Source: CAD feature listing. Evaluate the final solid. Frame: model axes, mm. A direction names the side the tool comes from. Round coordinates to 2 decimals unless told otherwise and drop trailing zeros. Loops run counter-clockwise (first coordinate to the right, second up) from the corner with the lowest first, then second, coordinate; pieces in that order, holes last.
(1) Section B-B, the plane x = 0. Return the cut outline in (y, z).
(2) Section D-D, the plane y = 20. Return the cut outline in (x, z), plus the area to 3 significant figures.
(3) Set-up query: faces 4 (the flat face through (49, -1, 15)), 5 (the cylindrical face through (48.85, -0.7, 1.57)). Return all of +Z, -Z, +X, -X, +Y, -Y with unobstructed straight access to the full face (end or side cutting, diameter ignored); none if empty.
(4) Section C-C, the plane y = -33. Return the cut outline in (x, z).
(5) Mould query, pull axis Y, two halves, no side actions, for faces 1 (the flat face through (-1, 1, 1.5)), 2 (the flat face through (0, -50, 1)), 3 (the cylindrical face through (0.65, -35.93, 0.74)). Classes: pulls with the +Y half, pulls with the -Y half, needs draft (parallel to the pull), parting line crosses it, or undercut.
(6) First-contact query: pin 1 Ø8 at (x, y) = (0, -33) entering from +Z. Flat tip, straight axial feed; report the tip coordinate or a pass-through.
(7) Material intervals for probe 1 along Y at (x, z) = (0, 0.6); probe 2 along X at (y, z) = (-10.5, 14); probe 3 along Z at (x, y) = (-2, 24), sorted ascending.
(8) Section A-A, the plane z = 20.5. Return the cut outline in (x, y).
```python
from build123d import *

# Parameters (mm, degrees)
SKETCH1_W                = 90
SKETCH1_H                = 100
BOSS_EXTRUDE1_DEPTH      = 10
CONVERT_SOLID1_START     = 1.5
CONVERT_SOLID1_OUTLINE_W = 90
CONVERT_SOLID1_OUTLINE_H = 100
CONVERT_SOLID1_DEPTH     = 8.5
EDGE_FLANGE1_DEPTH       = 100
EDGE_FLANGE2_DEPTH       = 100
SKETCH12_R               = 3
CUT_EXTRUDE1_DEPTH       = 75.849849699


# Read off the part's stored shape, not the designer's step: Convert-Solid1
# Sheet-metal steps are written as plain solids
with BuildPart() as part:
    # Sketch1 → Boss-Extrude1 (new body)
    with BuildSketch(Plane.XY):
        Rectangle(SKETCH1_W, SKETCH1_H)
    extrude(amount=BOSS_EXTRUDE1_DEPTH)

    # Convert-Solid1 outline → Convert-Solid1 (cut)
    with BuildSketch(Plane.XY.offset(CONVERT_SOLID1_START)):
        Rectangle(CONVERT_SOLID1_OUTLINE_W, CONVERT_SOLID1_OUTLINE_H)
    extrude(amount=CONVERT_SOLID1_DEPTH, mode=Mode.SUBTRACT)

    # Edge-Flange1 section (across the edge) → Edge-Flange1 (add)
    with BuildSketch(Plane(origin=(-49, 50, 1.5), x_dir=(1, 0, 0), z_dir=(0, -1, 0))):
        with BuildLine():
            Line((-1.5, 4), (-1.5, 22))
            Line((-1.5, 22), (0, 22))
            Line((0, 22), (0, 4))
            ThreePointArc((0, 4), (1.171572875, 1.171572875), (4, 0))
            Line((4, 0), (4, -1.5))
            ThreePointArc((4, -1.5), (0.110912703, 0.110912703), (-1.5, 4))
        make_face()
    extrude(amount=EDGE_FLANGE1_DEPTH)

    # Edge-Flange2 section (across the edge) → Edge-Flange2 (add)
    with BuildSketch(Plane(origin=(49, -50, 1.5), x_dir=(-1, 0, 0), z_dir=(0, 1, 0))):
        with BuildLine():
            Line((-1.5, 4), (-1.5, 22))
            Line((-1.5, 22), (0, 22))
            Line((0, 22), (0, 4))
            ThreePointArc((0, 4), (1.171572875, 1.171572875), (4, 0))
            Line((4, 0), (4, -1.5))
            ThreePointArc((4, -1.5), (0.110912703, 0.110912703), (-1.5, 4))
        make_face()
    extrude(amount=EDGE_FLANGE2_DEPTH)

    # Sketch12 → Cut-Extrude1 (cut, through all)
    with BuildSketch(Plane(origin=(0, 0, 0), x_dir=(-1, 0, 0), z_dir=(0, 0, -1))):
        with Locations((0, 33)):
            Circle(SKETCH12_R)
        with Locations((0, -33)):
            Circle(SKETCH12_R)
    extrude(amount=-CUT_EXTRUDE1_DEPTH, mode=Mode.SUBTRACT)


solid = part.part
```
Output values:
1. outline: (-50, 0) - (-36, 0) - (-36, 1.5) - (-50, 1.5) - close; (-30, 0) - (30, 0) - (30, 1.5) - (-30, 1.5) - close; (36, 0) - (50, 0) - (50, 1.5) - (36, 1.5) - close
2. outline: (-50.5, 5.5) arc R5.5 ccw to (-45, 0) - (45, 0) arc R5.5 ccw to (50.5, 5.5) - (50.5, 23.5) - (49, 23.5) - (49, 5.5) arc R4 cw to (45, 1.5) - (-45, 1.5) arc R4 cw to (-49, 5.5) - (-49, 23.5) - (-50.5, 23.5) - close
2. area: 211 mm2
3. face 4: +Z, +Y, -Y
3. face 5: -Z, +X, +Y, -Y
4. outline: (-50.5, 5.5) arc R5.5 ccw to (-45, 0) - (-3, 0) - (-3, 1.5) - (-45, 1.5) arc R4 cw to (-49, 5.5) - (-49, 23.5) - (-50.5, 23.5) - close; (3, 0) - (45, 0) arc R5.5 ccw to (50.5, 5.5) - (50.5, 23.5) - (49, 23.5) - (49, 5.5) arc R4 cw to (45, 1.5) - (3, 1.5) - close
5. face 1: needs draft
5. face 2: pulls with the -Y half
5. face 3: undercut
6. pin 1: stops at z = 1.5
7. probe 1: y = -50 to -36, -30 to 30, 36 to 50
7. probe 2: x = -50.5 to -49, 49 to 50.5
7. probe 3: z = 0 to 1.5
8. outline: (-50.5, -50) - (-49, -50) - (-49, 50) - (-50.5, 50) - close; (49, -50) - (50.5, -50) - (50.5, 50) - (49, 50) - close
